Check sheet for the modelled part. Datum: model origin and axes. Units: mm. Face numbers are marked on the shaded views. A direction names the side the tool comes from. Coordinates: 2 decimals unless noted, no trailing zeros. Loops run counter-clockwise (first coordinate to the right, second up) from the corner with the lowest first, then second, coordinate; pieces in that order, holes last. Notation, with made-up numbers: (-20.75, -14.75) -> (-1.75, -14.75) arc R34 cw to (-1.75, 24.25) -> close; hole circle Ø5 at (51, 0). An arc over 180 degrees is marked (long way). Use one line per item in the form item = value.
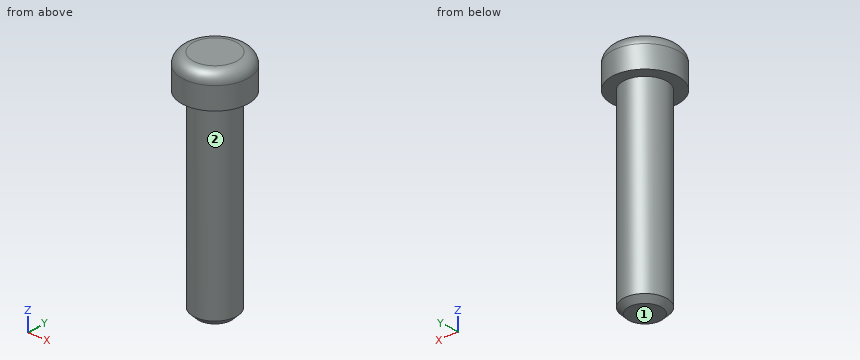
from build123d import *

# Parameters (mm, degrees)
F0_R     = 5.0038
F1_DEPTH = 44.45
F2_R     = 7.62
F2_R_2   = 5.0038
F3_DEPTH = 7.62
F4_R     = 2.54
F5_SIZE  = 1.27


with BuildPart() as f1:
    # F0 (on Top) → F1 (new body)
    with BuildSketch(Plane.XY):
        Circle(F0_R)
    extrude(amount=F1_DEPTH)

    # F2 (on face) → F3 (join)
    with BuildSketch(Plane.XY.offset(44.45)):
        Circle(F2_R)
        Circle(F2_R_2, mode=Mode.SUBTRACT)
        Circle(F2_R_2)
    extrude(amount=F3_DEPTH)

    # F4
    f4_edges = [f1.edges().sort_by_distance(p)[0] for p in [
        (-7.62, 0, 52.07),
    ]]
    fillet(f4_edges, radius=F4_R)

    # F5
    f5_edges = [f1.edges().sort_by_distance(p)[0] for p in [
        (-5.0038, 0, 0),
    ]]
    chamfer(f5_edges, length=F5_SIZE)


solid = f1.part
(1) Section check A-A, the plane y = 0. Record the boundary of the cut face in (x, z), plus the area to 3 significant figures.
Established:
outline = (-7.62, 44.45) -> (-5, 44.45) -> (-5, 1.27) -> (-3.73, 0) -> (3.73, 0) -> (5, 1.27) -> (5, 44.45) -> (7.62, 44.45) -> (7.62, 49.53) arc R2.54 ccw to (5.08, 52.07) -> (-5.08, 52.07) arc R2.54 ccw to (-7.62, 49.53) -> close
area = 557 mm²
(2) Go/stop test with flat-tipped pins: P1, Ø3, axis at y = 5, z = 45, coming from the -X side; P2, Ø4, axis at y = -0.5, z = 24.5, coming from the +X side; P3, Ø2, axis at x = 0, y = 1, coming from the -Z side; P4, Ø6, axis at y = 4, z = 9.5, coming from the -X side. Record where each tip stops, or that it passes through.
Established:
P1 = -6.77
P2 = 5
P3 = 0
P4 = -4.9
(3) Tool access check on the marked faces 1 and 2. Record the directions out of +Z, -Z, +X, -X, +Y, -Y that give a thin tool (end or side, any length) a straight path to the whole face; none if there is none.
Established:
face_1 = -Z, +X, -X, +Y, -Y
face_2 = -Z
(4) Section check C-C, the plane z = 38.5. Record the boundary of the cut face in (x, y), plus the area to 3 significant figures.
Established:
outline = circle Ø10.01 at (0, 0)
area = 78.7 mm²
(5) Scan lines: line 1 along Y through (x, z) = (0.25, 43); line 2 along X through (y, z) = (-3.25, 5.5). Record each from-to range of solid material in increasing order.
Established:
line_1 = -5 to 5
line_2 = -3.8 to 3.8
